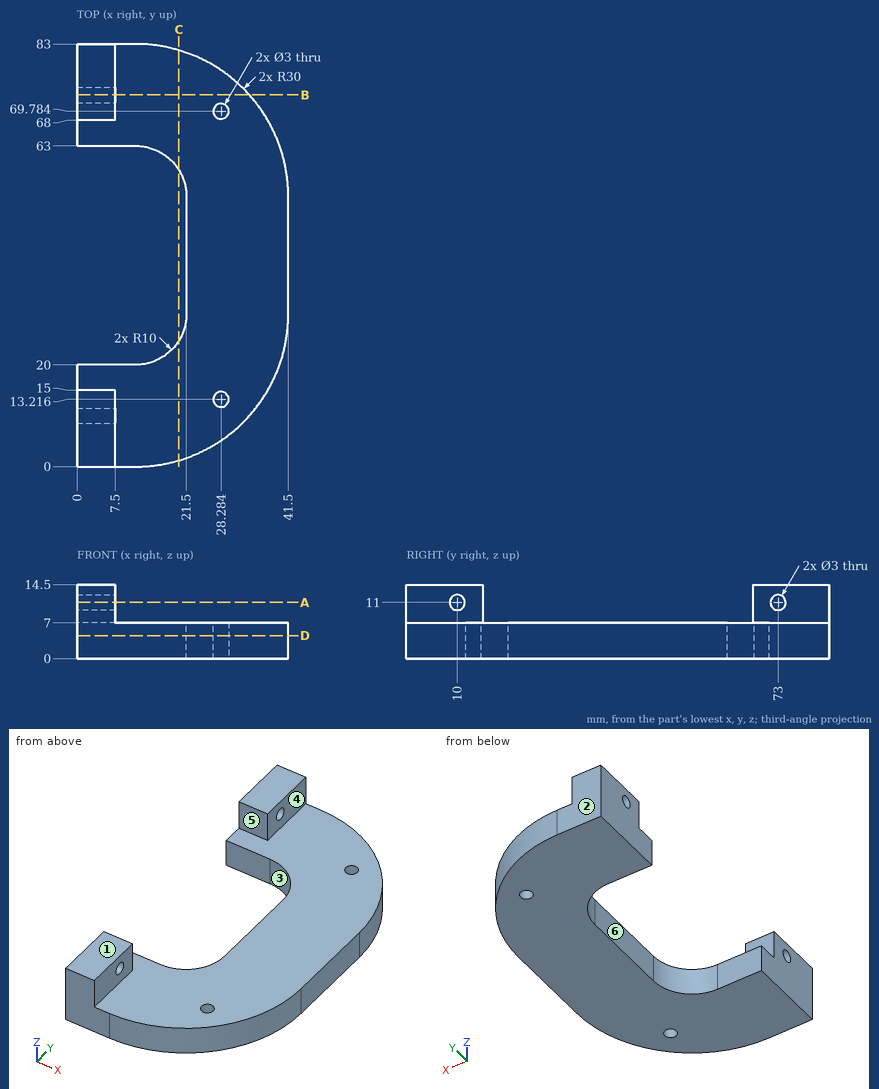
The figure shows three views and two pictorial views of one solid part (mm, origin at its lowest corner). Answer the questions. A direction names the side the tool comes from. Coordinates: 2 decimals unless noted, no trailing zeros. Order: outer loops, then holes, each group sorted by start corner. A loop starts at its lowest first (then second) coordinate and runs counter-clockwise, first axis right, second up.
Q1. A cutting plane is placed at C-C, the plane x = 20. Write down the section's boundary in (y, z).
Q2. For a pull along Y with two mould halves and no side action, classify the marked faces 1, 2 and 3 as pulls with the +Y half, pulls with the -Y half, needs draft (parallel to the pull), parting line crosses it, or undercut.
Q3. A cutting plane is placed at B-B, the plane y = 73. Write down the section's boundary in (x, z).
Q4. Consider line 1 (Y direction, x = 2, z = 11); line 2 (Y direction, x = 2, z = 3.5); line 3 (Y direction, x = 3, z = 10). Determine where each line is inside the solid, lowest interval first.
Q5. A cutting plane is placed at D-D, the plane z = 4.5. Write down the section's boundary in (x, y), and give its area (3 significant figures).
Q6. Which of the six approach directions +Z, -Z, +X, -X, +Y, -Y give full straight-line access (tool end or side, diameter ignored) to the marked faces 4, 5 and 6?
Q7. Given P1, Ø3.5, axis at y = 10, z = 11, coming from the +X side; P2, Ø2.5, axis at y = 73, z = 11, coming from the +X side; P3, Ø12.5, axis at x = 21.5, y = 39, coming from the +Z side; P4, Ø4, axis at x = 36, z = 4, coming from the -Y side, each flat-ended and moving along its own axis, determine where each tip first touches the part or whether it passes through.
Q8. A cutting plane is placed at A-A, the plane z = 11. Write down the section's boundary in (x, y), and give its area (3 significant figures).
Answers follow:
1. outline: (1.23, 0) - (24.73, 0) - (24.73, 7) - (1.23, 7) - close; (58.27, 0) - (81.77, 0) - (81.77, 7) - (58.27, 7) - close
2. face 1: needs draft
2. face 2: pulls with the +Y half
2. face 3: undercut
3. outline: (0, 0) - (33.86, 0) - (33.86, 7) - (7.5, 7) - (7.5, 9.5) - (0, 9.5) - close; (0, 12.5) - (7.5, 12.5) - (7.5, 14.5) - (0, 14.5) - close
4. line 1: y = 0 to 8.5, 11.5 to 15, 68 to 71.5, 74.5 to 83
4. line 2: y = 0 to 20, 63 to 83
4. line 3: y = 0 to 8.88, 11.12 to 15, 68 to 71.88, 74.12 to 83
5. outline: (0, 0) - (11.5, 0) arc R30 ccw to (41.5, 30) - (41.5, 53) arc R30 ccw to (11.5, 83) - (0, 83) - (0, 63) - (11.5, 63) arc R10 cw to (21.5, 53) - (21.5, 30) arc R10 cw to (11.5, 20) - (0, 20) - close; hole circle Ø3 at (28.28, 13.22); hole circle Ø3 at (28.28, 69.78)
5. area: 2,160 mm2
6. face 4: +Z, +X, +Y, -Y
6. face 5: +Z, +X, -X
6. face 6: +Z, -Z, -X
7. P1: stops at x = 7.5
7. P2: passes through
7. P3: stops at z = 7
7. P4: stops at y = 10.16
8. outline: (0, 0) - (7.5, 0) - (7.5, 8.5) - (0, 8.5) - close; (0, 11.5) - (7.5, 11.5) - (7.5, 15) - (0, 15) - close; (0, 68) - (7.5, 68) - (7.5, 71.5) - (0, 71.5) - close; (0, 74.5) - (7.5, 74.5) - (7.5, 83) - (0, 83) - close
8. area: 180 mm2
